```python
from build123d import *

# Parameters (mm, degrees)
EXTRUDE_1_DEPTH             = 10
HOLE_WIZARD_M41_D           = 4.5
HOLE_WIZARD_M41_CBORE_D     = 8
HOLE_WIZARD_M41_CBORE_DEPTH = 4
FILLET_1_R                  = 2
FILLET_2_R                  = 5
CHAMFER_1_SIZE              = 0.5


with BuildPart() as part:
    # Эскиз1 → Бобышка-Вытянуть1 (new body)
    with BuildSketch(Plane(origin=(0, 0, 0), x_dir=(1, 0, 0), z_dir=(0, 1, 0))):
        with BuildLine():
            Line((-3.5, -7.193747285), (-3.5, -21))
            Line((-3.5, -21), (3.5, -21))
            Line((3.5, -21), (3.5, -7.193747285))
            ThreePointArc((3.5, -7.193747285), (0, 8), (-3.5, -7.193747285))
        make_face()
    extrude(amount=EXTRUDE_1_DEPTH)

    # Цековка для винта с внутренним шестигранником M41 (through all)
    with Locations(Plane(origin=(0, 10, 0), x_dir=(1, 0, 0), z_dir=(0, 1, 0))):
        with Locations((0, 0)):
            CounterBoreHole(HOLE_WIZARD_M41_D / 2, HOLE_WIZARD_M41_CBORE_D / 2, HOLE_WIZARD_M41_CBORE_DEPTH)

    # Скругление1
    fillet_1_edges = [part.edges().sort_by_distance(p)[0] for p in [
        (3.5, 5, 21),
        (-3.5, 5, 21),
    ]]
    fillet(fillet_1_edges, radius=FILLET_1_R)

    # Скругление2
    fillet_2_edges = [part.edges().sort_by_distance(p)[0] for p in [
        (-3.5, 5, 7.193747285),
        (3.5, 5, 7.193747285),
    ]]
    fillet(fillet_2_edges, radius=FILLET_2_R)

    # Фаска1
    chamfer_1_edges = [part.edges().sort_by_distance(p)[0] for p in [
        (-4, 10, 0),
        (2.25, 0, 0),
        (3.5, 0, 14.418078893),
        (3.5, 10, 14.418078893),
        (0, 0, 21),
        (-2.914213562, 0, 20.414213562),
        (2.914213562, 0, 20.414213562),
        (0, 10, 21),
        (-2.914213562, 10, 20.414213562),
        (2.914213562, 10, 20.414213562),
        (0, 0, -8),
        (0, 10, -8),
        (-3.5, 0, 14.418078893),
        (-3.5, 10, 14.418078893),
        (3.953234455, 0, 7.756032051),
        (3.953234455, 10, 7.756032051),
        (-3.953234455, 0, 7.756032051),
        (-3.953234455, 10, 7.756032051),
    ]]
    chamfer(chamfer_1_edges, length=CHAMFER_1_SIZE)


solid = part.part
```
Part model, mm, in its own coordinate system. A direction names the side the tool comes from. Round coordinates to 2 decimals unless told otherwise and drop trailing zeros. Order: outer loops, then holes, each group sorted by start corner. A loop starts at its lowest first (then second) coordinate and runs counter-clockwise, first axis right, second up. Notation, with made-up numbers: M 31,14 L 69,14 A9 cw 69,21 Z; hole C -35,56.5 d4. An arc over 180 degrees is marked long. Put each result on its own line as item: value. Start each with the question number.
1. Tool access for faces 4 (the face through (0, 5, 21)), 5 (the face through (2, 6, 2)), 6 (the face through (3.5, 5, 14)): list every direction of +Z, -Z, +X, -X, +Y, -Y with a clear straight run to the whole face (end or side of a thin tool).
2. Two-plate mould, pull along X, no slides. Class faces 1 (the face through (-0.867, 7.774, 3.905)), 2 (the face through (-2.67, 0.14, 20.15)), 3 (the face through (3.966, 5.063, 7.729)): +X half, -X half, draft (parallel to the pull), parting line (faces both ways), or undercut.
3. Slice it at A-A on x = 0. List the corners of the cut face in (y, z), then the cut area to 3 significant figures.
4. Drop flat-ended pins along their axis: pin 1 (4.5 mm diameter, centred on y = 3, z = 13, fed in from -X); pin 2 (5 mm diameter, centred on x = 0, z = 0, fed in from +Y); pin 3 (4 mm diameter, centred on x = 0, z = 0, fed in from +Y); pin 4 (2.5 mm diameter, centred on y = 5.5, z = 13, fed in from +X). Give the stop position or say it passes through.
5. Drill centre lines: probe 1 along X at (y, z) = (4.5, 0); probe 2 along X at (y, z) = (7.95, 0); probe 3 along X at (y, z) = (8.5, 11.5). Where is each one in solid material? Low to high. Write a range as [from, to].
6. Slice it at B-B on y = 8.25. List the corners of the cut face in (x, z), then the cut area to 3 significant figures.
7. Slice it at C-C on z = 0. List the corners of the cut face in (x, y).
Findings:
1. face 4: +Z, +X, -X, +Y, -Y
1. face 5: +Y
1. face 6: +Z, +X, +Y, -Y
2. face 1: undercut
2. face 2: -X half
2. face 3: +X half
3. outline: M 0,-7.5 L 0.5,-8 L 9.5,-8 L 10,-7.5 L 10,-4.5 L 9.5,-4 L 6,-4 L 6,-2.25 L 0.5,-2.25 L 0,-2.75 Z; M 0,2.75 L 0.5,2.25 L 6,2.25 L 6,4 L 9.5,4 L 10,4.5 L 10,20.5 L 9.5,21 L 0.5,21 L 0,20.5 Z
3. area: 230 mm2
4. pin 1: x = -3.5
4. pin 2: y = 6
4. pin 3: through
4. pin 4: x = 3.5
5. probe 1: [-8, -2.25], [2.25, 8]
5. probe 2: [-8, -4], [4, 8]
5. probe 3: [-3.5, 3.5]
6. outline: M -5.23,6.05 A8 ccw long 5.23,6.05 A5 cw 3.5,9.84 L 3.5,19 A2 ccw 1.5,21 L -1.5,21 A2 ccw -3.5,19 L -3.5,9.84 A5 cw Z; hole C 0,0 d8
6. area: 244 mm2
7. outline: M -8,0.5 L -7.5,0 L -2.75,0 L -2.25,0.5 L -2.25,6 L -4,6 L -4,9.5 L -4.5,10 L -7.5,10 L -8,9.5 Z; M 2.25,0.5 L 2.75,0 L 7.5,0 L 8,0.5 L 8,9.5 L 7.5,10 L 4.5,10 L 4,9.5 L 4,6 L 2.25,6 Z
